```python
from build123d import *

# Parameters (mm, degrees)
SKETCH_1_W                   = 80
SKETCH_1_H                   = 14.999999944
SKETCH_1_H_2                 = 50
SKETCH_1_W_2                 = 14.999999944
SKETCH_1_W_3                 = 15.000000056
EXTRUDE_1_DEPTH              = 8
AXISHOLE_REACH               = 70.476
SKETCH_2_R                   = 10
LOCKINGSLOT_REACH            = 70.476
ADJUSTSLOT_REACH             = 70.476
FILLET_1_R                   = 2
HOLE_START                   = -39.999999944
HOLE_WIZARD_M4_1_OUTLINE_R   = 1.65
HOLE_WIZARD_M4_1_DEPTH       = 16.797680198
HOLE_WIZARD_M3_1_D           = 3.4
HOLE_WIZARD_M3_1_CSINK_D     = 6.72
HOLE_WIZARD_M3_1_CSINK_ANGLE = 90


# Read off the part's stored shape, not the designer's step: M4 나사 구멍1
with BuildPart() as part:
    # 스케치1 → 보스-돌출1 (new body)
    with BuildSketch(Plane.XY):
        with Locations((-5.6e-08, -32.499999972)):
            Rectangle(SKETCH_1_W, SKETCH_1_H)
        with Locations((-5.6e-08, 0)):
            Rectangle(SKETCH_1_W, SKETCH_1_H_2)
        Polygon((39.999999944, 39.999999832), (-40.000000056, 40.000000056), (-40.000000056, 25), (39.999999944, 25), align=None)
        with Locations((47.499999916, 0)):
            Rectangle(SKETCH_1_W_2, SKETCH_1_H_2)
        with Locations((-47.500000084, 0)):
            Rectangle(SKETCH_1_W_3, SKETCH_1_H_2)
        Polygon((-40.000000056, -25), (-55.000000112, -25), (-40.000000056, -39.999999944), align=None)
        Polygon((54.999999888, -25), (39.999999944, -25), (39.999999944, -39.999999944), align=None)
        Polygon((54.999999888, 25), (39.999999944, 39.999999832), (39.999999944, 25), align=None)
        Polygon((-40.000000056, 25), (-40.000000056, 40.000000056), (-55.000000112, 25), align=None)
    extrude(amount=EXTRUDE_1_DEPTH)

    # 스케치2 → AXISHOLE (cut, up to next)
    with BuildSketch(Plane.XY.offset(8), mode=Mode.PRIVATE) as axishole_sk1:
        Circle(SKETCH_2_R)
    axishole_tool1 = extrude(axishole_sk1.sketch, amount=-AXISHOLE_REACH, mode=Mode.PRIVATE) & part.part
    add(axishole_tool1.solids().sort_by_distance((0, 0, 8))[0], mode=Mode.SUBTRACT)

    # 스케치3 → LOCKINGSLOT (cut, up to next)
    with BuildSketch(Plane.XY.offset(8), mode=Mode.PRIVATE) as lockingslot_sk1:
        with BuildLine():
            ThreePointArc((-9.64100943, -35.980737029), (0, -37.25), (9.64100943, -35.980737029))
            ThreePointArc((9.64100943, -35.980737029), (11.231999688, -33.225061069), (8.476323727, -31.634070811))
            ThreePointArc((8.476323727, -31.634070811), (0, -32.75), (-8.476323727, -31.634070811))
            ThreePointArc((-8.476323727, -31.634070811), (-11.231999688, -33.225061069), (-9.64100943, -35.980737029))
        make_face()
    lockingslot_tool1 = extrude(lockingslot_sk1.sketch, amount=-LOCKINGSLOT_REACH, mode=Mode.PRIVATE) & part.part
    # 스케치3 → LOCKINGSLOT (cut, up to next)
    with BuildSketch(Plane.XY.offset(8), mode=Mode.PRIVATE) as lockingslot_sk2:
        with BuildLine():
            ThreePointArc((9.64100943, 35.980737029), (0, 37.25), (-9.64100943, 35.980737029))
            ThreePointArc((-9.64100943, 35.980737029), (-11.231999688, 33.225061069), (-8.476323727, 31.634070811))
            ThreePointArc((-8.476323727, 31.634070811), (0, 32.75), (8.476323727, 31.634070811))
            ThreePointArc((8.476323727, 31.634070811), (11.231999688, 33.225061069), (9.64100943, 35.980737029))
        make_face()
    lockingslot_tool2 = extrude(lockingslot_sk2.sketch, amount=-LOCKINGSLOT_REACH, mode=Mode.PRIVATE) & part.part
    add(lockingslot_tool1.solids().sort_by_distance((0, -34.473161, 8))[0], mode=Mode.SUBTRACT)
    add(lockingslot_tool2.solids().sort_by_distance((0, 34.473161, 8))[0], mode=Mode.SUBTRACT)

    # 스케치4 → ADJUSTSLOT (cut, up to next)
    with BuildSketch(Plane.XY.offset(8), mode=Mode.PRIVATE) as adjustslot_sk1:
        with BuildLine():
            Line((24.748737262, 24.748737262), (14.142135545, 14.142135545))
            ThreePointArc((14.142135545, 14.142135545), (19.999999888, 0), (14.142135545, -14.142135545))
            Line((14.142135545, -14.142135545), (24.748737262, -24.748737262))
            ThreePointArc((24.748737262, -24.748737262), (34.999999888, 0), (24.748737262, 24.748737262))
        make_face()
    adjustslot_tool1 = extrude(adjustslot_sk1.sketch, amount=-ADJUSTSLOT_REACH, mode=Mode.PRIVATE) & part.part
    add(adjustslot_tool1.solids().sort_by_distance((25.372551, 0, 8))[0], mode=Mode.SUBTRACT)

    # 필렛1
    fillet_1_edges = [part.edges().sort_by_distance(p)[0] for p in [
        (24.748737262, 24.748737262, 4),
        (24.748737262, -24.748737262, 4),
        (14.142135545, -14.142135545, 4),
        (14.142135545, 14.142135545, 4),
    ]]
    fillet(fillet_1_edges, radius=FILLET_1_R)

    # M4 나사 구멍1 outline → M4 나사 구멍1 (cut)
    with BuildSketch(Plane(origin=(0, 0, 0), x_dir=(1, 0, 0), z_dir=(0, 1, 0)).offset(HOLE_START)):
        with Locations((24.999999888, -4)):
            Circle(HOLE_WIZARD_M4_1_OUTLINE_R)
    hole_wizard_m4_1 = extrude(amount=HOLE_WIZARD_M4_1_DEPTH, mode=Mode.SUBTRACT)

    # 대칭 복사1: M4 나사 구멍1 across plane
    add(hole_wizard_m4_1.mirror(Plane(origin=(0, 0, 0), x_dir=(0, 0, 1), z_dir=(-1.3990850145084723e-09, -1.0, 0))), mode=Mode.SUBTRACT)

    # M3 육각 소켓 접시 머리 캡 나사용 카운터싱크1 (through all)
    with Locations(Plane(origin=(0, 0, 0), x_dir=(-1, 0, 0), z_dir=(0, 0, -1))):
        with Locations((51.000000112, -13), (51.000000112, 13), (-51.000000112, -13), (-51.000000112, 13)):
            CounterSinkHole(HOLE_WIZARD_M3_1_D / 2, HOLE_WIZARD_M3_1_CSINK_D / 2, counter_sink_angle=HOLE_WIZARD_M3_1_CSINK_ANGLE)


solid = part.part
```
The listing builds one solid part. Answer for the finished solid, in the listing's coordinates (mm). A direction names the side the tool comes from. Coordinates: 2 decimals unless noted, no trailing zeros. Loops run counter-clockwise (first coordinate to the right, second up) from the corner with the lowest first, then second, coordinate; pieces in that order, holes last. Notation, with made-up numbers: (51, -17.75) - (59, -17.75) arc R29 ccw to (59, 15.25) - close; hole circle Ø2 at (-24, -25). An arc over 180 degrees is marked (long way). Use a Markdown table: item, result. Add a question column.
1) The part is cut by section C-C, the plane y = -28. Give the vertices of the cut face in (x, z), and give its area (3 significant figures).
2) The part is cut by section A-A, the plane y = 0. Give the vertices of the cut face in (x, z), and give its area (3 significant figures).
3) The part is cut by section D-D, the plane y = 19. Give the vertices of the cut face in (x, z), and give its area (3 significant figures).
4) Find the intervals of material crossed by line 1 (X direction, y = 1.5, z = 1.5); line 2 (X direction, y = -13, z = 6.25); line 3 (Y direction, x = -7, z = 5.5), in increasing order.
5) For faces 5 (the cylindrical face through (-0.12, 32.75, 4.06)), 6 (the flat face through (-13, 1, 0)), determine the directions among +Z, -Z, +X, -X, +Y, -Y from which every point of the face is accessible in a straight line to the end or side of a thin tool.
6) Given pin 1 (10 mm diameter, centred on x = 19, y = 7.5, fed in from +Z); pin 2 (1.5 mm diameter, centred on y = -30, z = 4.5, fed in from -X); pin 3 (4.5 mm diameter, centred on x = 51, y = -13, fed in from -Z), each flat-ended and moving along its own axis, determine where each tip first touches the part or whether it passes through.
7) The mould has two halves that part along X. Classify faces 1 (the cylindrical face through (-52.7, -12.93, 4.87)), 2 (the flat face through (1, 40, 4)), 3 (the cylindrical face through (-11.244, 33.273, 4.056)), 4 (the flat face through (-55, 0, 4)): released by +X, released by -X, zero draft, split by the parting line, or undercut.
8) The part is cut by section B-B, the plane x = 25. Give the vertices of the cut face in (y, z), and give its area (3 significant figures).
Here are the results:
| question | item | result |
|---|---|---|
| 1 | outline | (-52, 0) - (52, 0) - (52, 8) - (-52, 8) - close; hole circle Ø3.3 at (25, 4) |
| 1 | area | 823 mm^2 |
| 2 | outline | (-55, 0) - (-10, 0) - (-10, 8) - (-55, 8) - close; (10, 0) - (20, 0) - (20, 8) - (10, 8) - close; (35, 0) - (55, 0) - (55, 8) - (35, 8) - close |
| 2 | area | 600 mm^2 |
| 3 | outline | (-55, 0) - (19, 0) - (19, 8) - (-55, 8) - close; (29.39, 0) - (55, 0) - (55, 8) - (29.39, 8) - close |
| 3 | area | 797 mm^2 |
| 4 | line 1 | x = -55 to -9.89, 9.89 to 19.94, 34.97 to 55 |
| 4 | line 2 | x = -55 to -52.7, -49.3 to 15.22, 32.5 to 49.3, 52.7 to 55 |
| 4 | line 3 | y = -40 to -36.59, -31.99 to -7.14, 7.14 to 31.99, 36.59 to 40 |
| 5 | face 5 | +Z, -Z |
| 5 | face 6 | -Z, +X, -X, +Y, -Y |
| 6 | pin 1 | stops at z = 8 |
| 6 | pin 2 | stops at x = -50.75 |
| 6 | pin 3 | stops at z = 1.11 |
| 7 | face 1 | undercut |
| 7 | face 2 | zero draft |
| 7 | face 3 | undercut |
| 7 | face 4 | released by -X |
| 8 | outline | (-40, 0) - (-23.86, 0) - (-23.86, 2.35) - (-40, 2.35) - close; (-40, 5.65) - (-23.86, 5.65) - (-23.86, 8) - (-40, 8) - close; (23.86, 0) - (40, 0) - (40, 2.35) - (23.86, 2.35) - close; (23.86, 5.65) - (40, 5.65) - (40, 8) - (23.86, 8) - close |
| 8 | area | 152 mm^2 |
